from build123d import *

# Parameters (mm, degrees)
F0_W     = 56
F0_H     = 34
F1_DEPTH = 20
F3_D     = 5
F4_SIZE  = 5.08


with BuildPart() as f1:
    # F0 (on Front) → F1 (new body)
    with BuildSketch(Plane.XZ):
        with Locations((28, 17)):
            Rectangle(F0_W, F0_H)
    extrude(amount=F1_DEPTH)

    # F3 (through all)
    with Locations(Plane.XY.offset(34)):
        with Locations((23.244202, -10)):
            Hole(F3_D / 2)

    # F4
    f4_edges = [f1.edges().sort_by_distance(p)[0] for p in [
        (56, -10, 34),
    ]]
    chamfer(f4_edges, length=F4_SIZE)


solid = f1.part
Check sheet for the modelled part. Datum: model origin and axes. Units: mm. Give positions to 0.01 mm unless a question says otherwise; leave off trailing zeros. Loops run counter-clockwise (first coordinate to the right, second up) from the corner with the lowest first, then second, coordinate; pieces in that order, holes last. Notation, with made-up numbers: M -33,44 L 1,44 A26 cw 1,58 Z; hole C 41.25,30 d4. An arc over 180 degrees is marked long. Answer as a JSON object with one key per item and string values. Group by question number.
Q1. Cross-section at C-C on x = 52. Record the cut outline in (y, z), then the cut area to 3 significant figures.
Q2. Cross-section at D-D on z = 25. Record the cut outline in (x, y), then the cut area to 3 significant figures.
Q3. Cross-section at B-B on z = 30.5. Record the cut outline in (x, y).
Q4. Cross-section at A-A on y = -10. Record the cut outline in (x, z), then the cut area to 3 significant figures.
Q5. Material ranges on line 1 along Y through (x, z) = (23.5, 6.5); line 2 along Y through (x, z) = (21, 9); line 3 along X through (y, z) = (-10.5, 4.5), recorded low to high. Write a range as [from, to].
Q6. Release check for a two-part mould opening along Y. For faces 1 (the flat face through (56, -10, 14)), 2 (the cylindrical face through (22.091, -12.218, 16.762)), 3 (the flat face through (28, -20, 17)) record: released by +Y, released by -Y, zero draft, split by the parting line, or undercut.
Evaluation:
{
 "1": {"outline": "M -20,0 L 0,0 L 0,32.92 L -20,32.92 Z", "area": "658 mm2"},
 "2": {"outline": "M 0,-20 L 56,-20 L 56,0 L 0,0 Z; hole C 23.24,-10 d5", "area": "1,100 mm2"},
 "3": {"outline": "M 0,-20 L 54.42,-20 L 54.42,0 L 0,0 Z; hole C 23.24,-10 d5"},
 "4": {"outline": "M 0,0 L 20.74,0 L 20.74,34 L 0,34 Z; M 25.74,0 L 56,0 L 56,28.92 L 50.92,34 L 25.74,34 Z", "area": "1,720 mm2"},
 "5": {"line 1": "y = [-20, -12.49], [-7.51, 0]", "line 2": "y = [-20, -11.1], [-8.9, 0]", "line 3": "x = [0, 20.79], [25.69, 56]"},
 "6": {"face 1": "zero draft", "face 2": "undercut", "face 3": "released by -Y"}
}
